Source: CAD feature listing. Evaluate the final solid. Frame: model axes, mm. Face numbers are marked on the shaded views. Coordinates: 2 decimals unless noted, no trailing zeros. Write each loop counter-clockwise with the first axis right and the second up, starting at its lowest first coordinate (ties: lowest second). Pieces come first, ordered by that corner, then holes. Notation, with made-up numbers: M -2,1 L 41,1 A19 cw 41,7 Z; hole C 83,3 d6. An arc over 180 degrees is marked long. Answer as CSV lines item,"result". Start each with the question number.
1. Section C-C on y = -2.5. Return the cut outline in (x, z), plus the area to 3 significant figures.
2. Section A-A on y = 3.25. Return the cut outline in (x, z), plus the area to 3 significant figures.
3. Mould query, pull axis X, two halves, no side actions, for the marked faces 1, 2 and 3. Classes: pulls with the +X half, pulls with the -X half, needs draft (parallel to the pull), parting line crosses it, or undercut.
4. Line query: probe 1 along Z at (x, y) = (5.5, -6); probe 2 along Y at (x, z) = (0, 11); probe 3 along X at (y, z) = (0.75, 7). Output: solid intervals per line, ascending. Write a range as [from, to].
5. Contact query for flat-ended pins moving along their axis: pin 1 Ø5 at (x, z) = (-4, 16.5) entering from +Y; pin 2 Ø6 at (y, z) = (1.5, 23) entering from -X; pin 3 Ø1.5 at (x, z) = (-2, 32.5) entering from +Y; pin 4 Ø7 at (x, y) = (0, 0) entering from +Z. Output: stop coordinate, or through.
6. Section B-B on z = 20. Return the cut outline in (x, y), plus the area to 3 significant figures.
```python
from build123d import *

# Parameters (mm, degrees)
SKETCH1_R               = 10
BOSS_EXTRUDE1_DEPTH     = 37
CUT_EXTRUDE1_DEPTH      = 10
CUT_EXTRUDE1_DEPTH_BACK = 40
SKETCH2_R               = 2
BOSS_EXTRUDE3_DEPTH     = 37
SKETCH4_R               = 4
CUT_EXTRUDE2_DEPTH      = 40
SKETCH6_W               = 33
SKETCH6_H               = 6.863237298


with BuildPart() as part:
    # Sketch1 → Boss-Extrude1 (new body)
    with BuildSketch(Plane.XY):
        Circle(SKETCH1_R)
    extrude(amount=BOSS_EXTRUDE1_DEPTH)

    # Sketch2 → Cut-Extrude1 (cut, two sides: drawn at the far end of the back side and taken through both)
    with BuildSketch(Plane.XY.offset(37).offset(-CUT_EXTRUDE1_DEPTH_BACK)):
        with Locations((0, 10)):
            Circle(SKETCH2_R)
        with Locations((4.067366431, 9.135454576)):
            Circle(SKETCH2_R)
        with Locations((7.431448255, 6.691306064)):
            Circle(SKETCH2_R)
        with Locations((9.510565163, 3.090169944)):
            Circle(SKETCH2_R)
        with Locations((9.945218954, -1.045284633)):
            Circle(SKETCH2_R)
        with Locations((8.660254038, -5)):
            Circle(SKETCH2_R)
        with Locations((5.877852523, -8.090169944)):
            Circle(SKETCH2_R)
        with Locations((2.079116908, -9.781476007)):
            Circle(SKETCH2_R)
        with Locations((-2.079116908, -9.781476007)):
            Circle(SKETCH2_R)
        with Locations((-5.877852523, -8.090169944)):
            Circle(SKETCH2_R)
        with Locations((-8.660254038, -5)):
            Circle(SKETCH2_R)
        with Locations((-9.945218954, -1.045284633)):
            Circle(SKETCH2_R)
        with Locations((-9.510565163, 3.090169944)):
            Circle(SKETCH2_R)
        with Locations((-7.431448255, 6.691306064)):
            Circle(SKETCH2_R)
        with Locations((-4.067366431, 9.135454576)):
            Circle(SKETCH2_R)
    extrude(amount=CUT_EXTRUDE1_DEPTH + CUT_EXTRUDE1_DEPTH_BACK, mode=Mode.SUBTRACT)

    # Sketch3 → Boss-Extrude3 (add)
    with BuildSketch(Plane.XY):
        with BuildLine():
            Line((2.168086595, 9.762141185), (1.989974874, 9.8))
            ThreePointArc((1.989974874, 9.8), (2.097960142, 9.870126453), (2.168086595, 9.762141185))
        make_face()
        with BuildLine():
            Line((5.951266195, 8.036319473), (5.803951609, 8.143349785))
            ThreePointArc((5.803951609, 8.143349785), (5.931124058, 8.163491922), (5.951266195, 8.036319473))
        make_face()
        with BuildLine():
            Line((8.705417805, 4.920945116), (8.614372384, 5.078640412))
            ThreePointArc((8.614372384, 5.078640412), (8.738742742, 5.045315475), (8.705417805, 4.920945116))
        make_face()
        with BuildLine():
            Line((9.95432359, 0.954694644), (9.935289914, 1.135787973))
            ThreePointArc((9.935289914, 1.135787973), (10.035353417, 1.054758147), (9.95432359, 0.954694644))
        make_face()
        with BuildLine():
            Line((9.482036394, -3.176631206), (9.538305559, -3.003452524))
            ThreePointArc((9.538305559, -3.003452524), (9.596760318, -3.118176447), (9.482036394, -3.176631206))
        make_face()
        with BuildLine():
            Line((7.370218964, -6.758688661), (7.49206152, -6.623368794))
            ThreePointArc((7.49206152, -6.623368794), (7.498800176, -6.751950006), (7.370218964, -6.758688661))
        make_face()
        with BuildLine():
            Line((3.984023719, -9.172107446), (4.150371981, -9.098044428))
            ThreePointArc((4.150371981, -9.098044428), (4.104229359, -9.218250068), (3.984023719, -9.172107446))
        make_face()
        with BuildLine():
            Line((-0.091045421, -9.999585528), (0.091045421, -9.999585528))
            ThreePointArc((0.091045421, -9.999585528), (0, -10.090630949), (-0.091045421, -9.999585528))
        make_face()
        with BuildLine():
            Line((-4.150371981, -9.098044428), (-3.984023719, -9.172107446))
            ThreePointArc((-3.984023719, -9.172107446), (-4.104229359, -9.218250068), (-4.150371981, -9.098044428))
        make_face()
        with BuildLine():
            Line((-7.49206152, -6.623368794), (-7.370218964, -6.758688661))
            ThreePointArc((-7.370218964, -6.758688661), (-7.498800176, -6.751950006), (-7.49206152, -6.623368794))
        make_face()
        with BuildLine():
            Line((-9.538305559, -3.003452524), (-9.482036394, -3.176631206))
            ThreePointArc((-9.482036394, -3.176631206), (-9.596760318, -3.118176447), (-9.538305559, -3.003452524))
        make_face()
        with BuildLine():
            Line((-9.935289914, 1.135787973), (-9.95432359, 0.954694644))
            ThreePointArc((-9.95432359, 0.954694644), (-10.035353417, 1.054758147), (-9.935289914, 1.135787973))
        make_face()
        with BuildLine():
            Line((-8.614372384, 5.078640412), (-8.705417805, 4.920945116))
            ThreePointArc((-8.705417805, 4.920945116), (-8.738742742, 5.045315475), (-8.614372384, 5.078640412))
        make_face()
        with BuildLine():
            Line((-5.803951609, 8.143349785), (-5.951266195, 8.036319473))
            ThreePointArc((-5.951266195, 8.036319473), (-5.931124058, 8.163491922), (-5.803951609, 8.143349785))
        make_face()
        with BuildLine():
            Line((-1.989974874, 9.8), (-2.168086595, 9.762141185))
            ThreePointArc((-2.168086595, 9.762141185), (-2.097960142, 9.870126453), (-1.989974874, 9.8))
        make_face()
    extrude(amount=BOSS_EXTRUDE3_DEPTH)

    # Sketch4 → Cut-Extrude2 (cut)
    with BuildSketch(Plane.XY.offset(37)):
        Circle(SKETCH4_R)
    extrude(amount=-CUT_EXTRUDE2_DEPTH, mode=Mode.SUBTRACT)

    # Sketch6 → Cut-Revolve7 (revolve, cut)
    with BuildSketch(Plane(origin=(0, 0, 0), x_dir=(0, 0, -1), z_dir=(1, 0, 0)), mode=Mode.PRIVATE) as cut_revolve7_sk:
        with Locations((-18.5, -9.431204177)):
            Rectangle(SKETCH6_W, SKETCH6_H)
    revolve(cut_revolve7_sk.sketch.rotate(Axis((0, 0, 10.741005804), (0, 0, 1)), 270), axis=Axis((0, 0, 10.741005804), (0, 0, 1)), mode=Mode.SUBTRACT)


solid = part.part
```
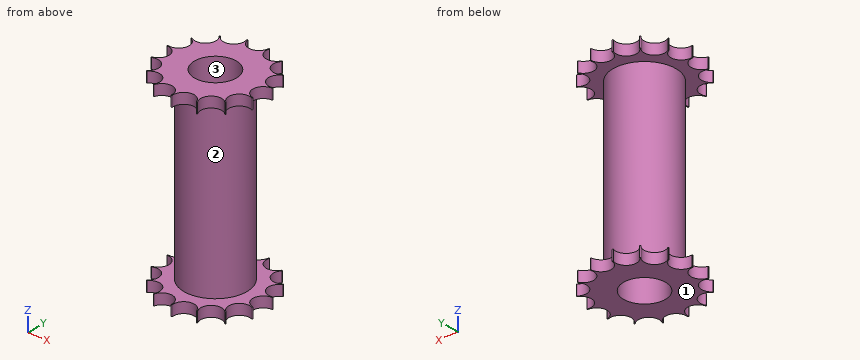
Values:
1,outline,"M -8.57,0 L -3.12,0 L -3.12,37 L -8.57,37 L -8.57,35 L -5.45,35 L -5.45,2 L -8.57,2 Z; M 3.12,0 L 8.57,0 L 8.57,2 L 5.45,2 L 5.45,35 L 8.57,35 L 8.57,37 L 3.12,37 Z"
1,area,"197 mm²"
2,outline,"M -7.52,0 L -2.33,0 L -2.33,37 L -7.52,37 L -7.52,35 L -5.04,35 L -5.04,2 L -7.52,2 Z; M 2.33,0 L 7.52,0 L 7.52,2 L 5.04,2 L 5.04,35 L 7.52,35 L 7.52,37 L 2.33,37 Z"
2,area,"220 mm²"
3,face 1,"needs draft"
3,face 2,"parting line crosses it"
3,face 3,"undercut"
4,probe 1,"[0, 2], [35, 37]"
4,probe 2,"[-6, -4], [4, 6]"
4,probe 3,"[-5.95, -3.93], [3.93, 5.95]"
5,pin 1,"y = 5.81"
5,pin 2,"x = -6"
5,pin 3,"y = 5.87"
5,pin 4,"through"
6,outline,"C 0,0 d12; hole C 0,0 d8"
6,area,"62.8 mm²"
